Source: CAD feature listing. Evaluate the final solid. Frame: model axes, mm. Face numbers are marked on the shaded views. A direction names the side the tool comes from. Coordinates: 2 decimals unless noted, no trailing zeros. Loops run counter-clockwise (first coordinate to the right, second up) from the corner with the lowest first, then second, coordinate; pieces in that order, holes last.
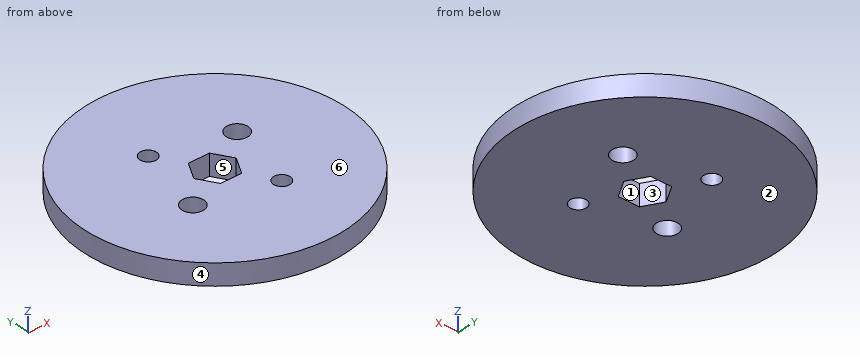
Autodesk Inventor part; units mm, degrees
ref_plane "YZ Plane" through (0, 0, 0) normal (1, 0, 0) x (0, 1, 0)
ref_plane "XZ Plane" through (0, 0, 0) normal (0, 1, 0) x (-1, 0, 0)
ref_plane "XY Plane" through (0, 0, 0) normal (0, 0, 1) x (1, 0, 0)
sketch "Sketch1" plane through (0, 0, 0) normal (0, 0, 1) x (1, 0, 0)
  circle A0 centre (0, 0) radius 27.6352
  dimension "d0" = 55.2704
extrude "Extrusion1" add sketch "Sketch1" along normal blind 3.175
sketch "Sketch2" plane through (0, 0, 3.175) normal (0, 0, 1) x (1, 0, 0)
  circle A0 centre (0, 0) radius 27.6352
  line L0 (0, 27.6352) -> (0, 0)
  line L1 (0, 0) -> (23.9328, -13.8176)
  line L2 (0, 0) -> (-23.9328, -13.8176)
  line L3 (0, 0) -> (27.6352, 0) construction
  line L4 (0, 27.6352) -> (0, 19.4152)
  line L5 (0, 19.4152) -> (5.08, 19.4152)
  line L6 (0, 19.4152) -> (-5.08, 19.4152)
  arc A1 (5.08, 19.4152) -> (-5.08, 19.4152) centre (0, -5.5937) ccw
  line L7 (-5.08, 19.4152) -> (2.5298, 19.4152) construction
  line L8 (-5.08, 19.4152) -> (-7.5281, 26.5901)
  line L9 (-5.08, 19.4152) -> (2.501, 19.4152) construction
  line L10 (5.08, 19.4152) -> (7.5281, 26.5901)
  line L11 (5.08, 19.4152) -> (12.661, 19.4152) construction
  line L12 (23.9328, -13.8176) -> (16.8277, -9.7155)
  line L13 (16.8277, -9.7155) -> (19.355, -5.3381)
  line L14 (16.8277, -9.7155) -> (14.3004, -14.0929)
  line L15 (16.8277, -9.7155) -> (17.2897, -9.9822)
  arc A2 (14.3004, -14.0929) -> (19.355, -5.3381) centre (-3.6819, 2.1257) ccw
  point P0 (0.3732, 19.9232)
  point P1 (0, 19.9259)
  dimension "d3" = 120
  dimension "d5" = 120
  dimension "d6" = 120
  dimension "d7" = 8.22
  dimension "d8" = 5.08
  dimension "d9" = 5.08
  dimension "d11" = 108.84
  dimension "d12" = 71.16
  dimension "d13" = 8.2042
  dimension "d14" = 5.0546
  dimension "d15" = 5.0546
  dimension "d16" = 6.16
  dimension "d17" = 0.5334
  dimension "d51" = 0.508
extrude "Extrusion2" cut sketch "Sketch2" against normal blind 3.175 contours L10 A1 L0 A0 | L0 A1 L8 A0
pattern_circular "Circular Pattern1" count 3 over 360 about axis through (0, 0, 0) along (0, 0, 1) of "Extrusion2"
sketch "Sketch4" plane through (0, 0, 3.175) normal (0, 0, 1) x (1, 0, 0)
  line L0 (-1.6129, -2.7686) -> (1.6129, -2.7686)
  line L1 (0, 2.7686) -> (0, 0)
  line L2 (0, -2.7686) -> (0, 0)
  line L3 (-1.6021, 2.7749) -> (1.6021, 2.7749)
  line L4 (1.6021, 2.7749) -> (3.2042, 0)
  line L5 (3.2042, 0) -> (1.6021, -2.7749)
  line L6 (1.6021, -2.7749) -> (-1.6021, -2.7749)
  line L7 (-1.6021, -2.7749) -> (-3.2042, 0)
  line L8 (-3.2042, 0) -> (-1.6021, 2.7749)
  line L9 (0, 0) -> (6.3283, 0)
extrude "Extrusion3" cut sketch "Sketch4" against normal blind 25.4
sketch "Sketch5" plane through (0, 0, 3.175) normal (0, 0, 1) x (1, 0, 0)
  line L0 (0, 0) -> (-11.9711, 20.5846)
  line L1 (-5.08, 19.4152) -> (-7.5281, 26.5901)
  circle A0 centre (-11.9711, 20.5846) radius 2.159
  line L2 (0, 0) -> (11.8412, 20.6596)
  line L3 (7.5281, 26.5901) -> (5.08, 19.4152)
  circle A1 centre (11.8412, 20.6596) radius 2.159
  line L4 (0, 0) -> (23.8124, 0.075)
  line L5 (19.3541, -5.3082) -> (26.7917, -6.7755)
  circle A2 centre (23.8124, 0.075) radius 2.159
  line L6 (0, 0) -> (11.9959, -20.5702)
  line L7 (19.2636, -19.8146) -> (14.2741, -14.107)
  circle A3 centre (11.9959, -20.5702) radius 2.159
  line L8 (0, 0) -> (-11.8291, -20.6666)
  line L9 (-14.2741, -14.107) -> (-19.2636, -19.8146)
  circle A4 centre (-11.8291, -20.6666) radius 2.159
  line L10 (-19.3541, -5.3082) -> (-26.7917, -6.7755)
  line L11 (0, 0) -> (-23.7488, -0.1036)
  line L12 (0, 0) -> (23.749, 0) construction
  dimension "d52" = 23.8125
  dimension "d54" = 4.318
  dimension "d55" = 23.8125
  dimension "d57" = 4.318
  dimension "d58" = 23.8125
  dimension "d60" = 4.318
  dimension "d61" = 23.8125
  dimension "d63" = 4.318
  dimension "d64" = 23.8125
  dimension "d66" = 4.318
  dimension "d69" = 23.8125
  dimension "d70" = 23.8252
  dimension "d82" = 5.969
  dimension "d86" = 59.931
  dimension "d88" = 23.749
  dimension "d89" = 180.25
extrude "Extrusion4" cut sketch "Sketch5" against normal blind 25.4
hole "Hole2" at (-23.7488, -0.1036, 3.175) direction (0, 0, -1) diameter 4.318 depth 25.4 tip angle 118
sketch "Sketch7" plane through (0, 0, 3.175) normal (0, 0, 1) x (1, 0, 0)
  line L0 (1.6021, 2.7749) -> (3.2042, 0)
  line L1 (2.4031, 1.3874) -> (6.9025, 4.0082)
  line L2 (2.4031, 1.3874) -> (7.6101, 1.3874) construction
  circle A0 centre (6.9025, 4.0082) radius 1.6339
  point P0 (0, 0)
  dimension "d105" = 5.207
  dimension "d106" = 30.22
  dimension "d107" = 3.2677
extrude "Extrusion5" cut sketch "Sketch7" against normal blind 25.4
sketch "Sketch8" plane through (0, 0, 3.175) normal (0, 0, 1) x (1, 0, 0)
  line L0 (-3.2042, 0) -> (-1.6021, -2.7749)
  line L1 (-2.4031, -1.3874) -> (-6.9023, -4.0085)
  circle A0 centre (-6.9023, -4.0085) radius 1.6339
  point P0 (0, 0)
  dimension "d112" = 5.207
  dimension "d113" = 3.2677
extrude "Extrusion6" cut sketch "Sketch8" against normal blind 25.4
thicken "Thicken1" operation add thickness 0.635 both sides no extend neighbours yes toward (-0.946424, -0.3229265, 0) faces at (-6.7121, 24.1984, 1.0583)
thicken "Thicken2" operation add thickness 0.635 both sides no extend neighbours yes toward (0.946424, -0.3229265, 0) faces at (5.896, 21.8068, 2.1167)
thicken "Thicken3" operation add thickness 0.635 both sides no extend neighbours yes toward (0.1935495, 0.9810905, 0) faces at (24.3125, -6.2864, 2.1167)
thicken "Thicken4" operation add thickness 0.635 both sides no extend neighbours yes toward (-0.7528746, -0.658164, 0) faces at (17.6004, -17.9121, 1.0583)
thicken "Thicken5" operation add thickness 0.635 both sides no extend neighbours yes toward (-0.1935495, 0.9810905, 0) faces at (-24.3125, -6.2864, 1.0583)
thicken "Thicken6" operation add thickness 0.635 both sides no extend neighbours yes toward (0.7528746, -0.658164, 0) faces at (-17.6004, -17.9121, 2.1167)
thicken "Thicken7" operation add thickness 0.381 both sides no extend neighbours yes toward (0.1744546, -0.9846652, 0) faces at (-4.452, 19.5346, 2.1167)
thicken "Thicken8" operation add thickness 0.381 both sides no extend neighbours yes toward (-0.9217033, 0.3878957, 0) faces at (18.6772, -7.1021, 1.0583)
thicken "Thicken9" operation add thickness 0.381 both sides no extend neighbours yes toward (0.7655178, 0.6434147, 0) faces at (-14.6914, -13.6229, 2.1167)
sketch "Sketch14" plane through (0, 0, 3.175) normal (0, 0, 1) x (1, 0, 0)
  line L0 (0, 0) -> (-4.0114, 6.9228)
  line L1 (0, 0) -> (8.001, 0) construction
  line L2 (0, 0) -> (4.0114, -6.9228)
  line L3 (0, 0) -> (8.001, 0) construction
  dimension "d170" = 8.001
  dimension "d171" = 120.09
  dimension "d172" = 8.001
  dimension "d173" = 59.91
hole "Hole5" at (-4.0114, 6.9228, 3.175) at (4.0114, -6.9228, 3.175) direction (0, 0, -1) diameter 2.4892 depth 9.525 tip angle 118
sketch "Sketch15" plane through (0, 0, 3.175) normal (0, 0, 1) x (1, 0, 0)
  circle A0 centre (0, 0) radius 19.5449
sketch "Sketch16" plane through (0, 0, 3.175) normal (0, 0, 1) x (1, 0, 0)
  circle A0 centre (0, 0) radius 27.6352
  circle A1 centre (0, 0) radius 19.5449
  arc A2 (-8.1376, 26.4099) -> (-26.9405, -6.1576) centre (0, 0) ccw
  arc A3 (26.9405, -6.1576) -> (8.1376, 26.4099) centre (0, 0) ccw
  arc A4 (-18.8029, -20.2523) -> (18.8029, -20.2523) centre (0, 0) ccw
  arc A5 (13.5925, -14.2922) -> (19.1737, -4.6254) centre (-4.8443, 2.7969) ccw
  arc A6 (-19.1737, -4.6254) -> (-13.5925, -14.2922) centre (4.8443, 2.7969) ccw
  arc A7 (5.5811, 18.9176) -> (-5.5811, 18.9176) centre (0, -5.5937) ccw
extrude "Extrusion9" cut sketch "Sketch16" against normal blind 25.4
equation "\"d55\" = d52"
equation "\"d58\" = d52"
equation "\"d61\" = d52"
equation "\"d64\" = d52"
equation "\"d69\" = d52"
properties part number "NewMechanumWheelHub"
Q1. Section query C-C on x = -9. Return the cut outline in (y, z) (3 decimals).
Q2. Draft query along X for the marked faces 1, 2, 3 and 4. Return one class per face: released by +X, released by -X, zero draft, split by the parting line, or undercut.
Q3. Reachability of the marked faces 5 and 6 from +Z, -Z, +X, -X, +Y, -Y: full face, straight path, thin tool, end or side. Return the list, or none.
Q4. Material intervals for line 1 along Y through (x, z) = (5, 1.7); line 2 along X through (y, z) = (-6, 0.85); line 3 along Y through (x, z) = (5.5, 2.3), sorted ascending.
Q5. Section query B-B on z = 0.8. Return the cut outline in (x, y).
Q6. Section query A-A on x = 0. Return the cut outline in (y, z) (3 decimals).
Q7. Section query D-D on y = 10.5. Return the cut outline in (x, z) (3 decimals), then the cut area to 3 significant figures.
Q8. First-contact query: pin 1 Ø1 at (x, z) = (-0.5, 1.5) entering from +Y; pin 2 Ø1.5 at (x, z) = (14, 1) entering from +Y; pin 3 Ø1 at (y, z) = (-5.5, 0.5) entering from +X. Flat tips, straight axial feed; report the tip coordinate or a pass-through.
Resolved:
1. outline: (-17.349, 0) - (17.349, 0) - (17.349, 3.175) - (-17.349, 3.175) - close
2. face 1: undercut
2. face 2: zero draft
2. face 3: undercut
2. face 4: split by the parting line
3. face 5: +Z, -Z
3. face 6: +Z, +X, -X, +Y, -Y
4. line 1: y = -18.89 to -7.68, -6.17 to 18.89
4. line 2: x = -18.6 to 3.18, 4.85 to 18.6
4. line 3: y = -18.76 to 3.17, 4.85 to 18.76
5. outline: circle Ø39.09 at (0, 0); hole circle Ø3.27 at (-6.9, -4.01); hole circle Ø2.49 at (-4.01, 6.92); hole (-3.2, 0) - (-1.6, -2.77) - (1.6, -2.77) - (3.2, 0) - (1.6, 2.77) - (-1.6, 2.77) - close; hole circle Ø2.49 at (4.01, -6.92); hole circle Ø3.27 at (6.9, 4.01)
6. outline: (-19.545, 0) - (-2.775, 0) - (-2.775, 3.175) - (-19.545, 3.175) - close; (2.775, 0) - (19.545, 0) - (19.545, 3.175) - (2.775, 3.175) - close
7. outline: (-16.485, 0) - (16.485, 0) - (16.485, 3.175) - (-16.485, 3.175) - close
7. area: 105 mm2
8. pin 1: stops at y = 19.54
8. pin 2: stops at y = 14.37
8. pin 3: stops at x = 18.89
